Check sheet for the modelled part. Datum: model origin and axes. Units: mm. Face numbers are marked on the shaded views. A direction names the side the tool comes from. Round coordinates to 2 decimals unless told otherwise and drop trailing zeros. Write each loop counter-clockwise with the first axis right and the second up, starting at its lowest first coordinate (ties: lowest second). Pieces come first, ordered by that corner, then holes. Notation, with made-up numbers: (72, -14) -> (101, -14) arc R32 cw to (101, 16) -> close; hole circle Ø11 at (-8, 35). An arc over 180 degrees is marked (long way). One line per item, written item: value.
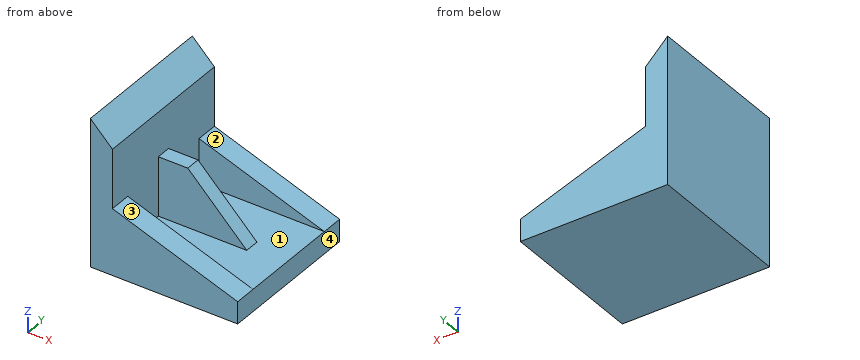
from build123d import *

# Parameters (mm, degrees)
F1_DEPTH = 127
F2_DEPTH = 12.7
F4_DEPTH = 38.1
F6_DEPTH = 38.1


with BuildPart() as f1:
    # F0 (on Front) → F1 (new body, symmetric)
    with BuildSketch(Plane.XZ):
        Polygon((0, 254), (0, 0), (254, 0), (254, 38.1), (190.5, 38.1), (38.1, 38.1), (38.1, 139.7), (38.1, 215.9), align=None)
    extrude(amount=F1_DEPTH, both=True)

    # F0 (on Front) → F2 (join, symmetric)
    with BuildSketch(Plane.XZ):
        Polygon((88.9, 139.7), (38.1, 139.7), (38.1, 38.1), (190.5, 38.1), align=None)
    extrude(amount=F2_DEPTH, both=True)

    # F3 (on face) → F4 (join)
    with BuildSketch(Plane.XZ.offset(127)):
        Polygon((254, 38.1), (38.1, 114.3), (38.1, 38.1), align=None)
    extrude(amount=-F4_DEPTH)

    # F5 (on face) → F6 (join)
    with BuildSketch(Plane(origin=(0, 127, 0), x_dir=(-1, 0, 0), z_dir=(0, 1, 0))):
        Polygon((-38.1, 38.1), (-38.1, 114.3), (-254, 38.1), align=None)
    extrude(amount=-F6_DEPTH)


solid = f1.part
Item 1: Sectioned sample at C-C (x = 100). Enter the section's corners in (y, z), then the cut area to 3 significant figures.
Result set:
outline: (-127, 0) -> (127, 0) -> (127, 92.45) -> (88.9, 92.45) -> (88.9, 38.1) -> (12.7, 38.1) -> (12.7, 128.6) -> (-12.7, 128.6) -> (-12.7, 38.1) -> (-88.9, 38.1) -> (-88.9, 92.45) -> (-127, 92.45) -> close
area: 16,100 mm^2
Item 2: Sectioned sample at D-D (y = 111.5). Enter the section's corners in (x, z), then the cut area to 3 significant figures.
Result set:
outline: (0, 0) -> (254, 0) -> (254, 38.1) -> (38.1, 114.3) -> (38.1, 215.9) -> (0, 254) -> close
area: 25,400 mm^2
Item 3: Sectioned sample at B-B (y = -1.5). Enter the section's corners in (x, z), then the cut area to 3 significant figures.
Result set:
outline: (0, 0) -> (254, 0) -> (254, 38.1) -> (190.5, 38.1) -> (88.9, 139.7) -> (38.1, 139.7) -> (38.1, 215.9) -> (0, 254) -> close
area: 27,500 mm^2
Item 4: Tool access check on the marked faces 1, 2, 3 and 4. Record the directions out of +Z, -Z, +X, -X, +Y, -Y that give a thin tool (end or side, any length) a straight path to the whole face; none if there is none.
Result set:
face 1: +Z, +X
face 2: +Z, +X, +Y
face 3: +Z, +X, -Y
face 4: +Z, -Z, +X, +Y, -Y
Item 5: Depth check by flat-ended pin: pin 1 (12 mm diameter, centred on x = 166, y = -43, fed in from -Z); pin 2 (8 mm diameter, centred on y = 27, z = 116.5, fed in from +X); pin 3 (7.5 mm diameter, centred on x = 61.5, y = 5, fed in from +Z). Enter the tip coordinate at first touch or a pass-through.
Result set:
pin 1: z = 0
pin 2: x = 38.1
pin 3: z = 139.7
Item 6: Sectioned sample at A-A (z = 85.5). Enter the section's corners in (x, y), then the cut area to 3 significant figures.
Result set:
outline: (0, -127) -> (119.7, -127) -> (119.7, -88.9) -> (38.1, -88.9) -> (38.1, -12.7) -> (143.1, -12.7) -> (143.1, 12.7) -> (38.1, 12.7) -> (38.1, 88.9) -> (119.7, 88.9) -> (119.7, 127) -> (0, 127) -> close
area: 18,600 mm^2
Item 7: Material ranges on line 1 along Y through (x, z) = (160.5, 43.5); line 2 along X through (y, z) = (27, 131), recorded low to high.
Result set:
line 1: -127 to -88.9, -12.7 to 12.7, 88.9 to 127
line 2: 0 to 38.1
